CAD build for the part. Positions are in the model's coordinates, mm. A direction names the side the tool comes from. Coordinates: 2 decimals unless noted, no trailing zeros. Order: outer loops, then holes, each group sorted by start corner. A loop starts at its lowest first (then second) coordinate and runs counter-clockwise, first axis right, second up. Notation, with made-up numbers: M 0.5,-14 L 21.5,-14 A29 ccw 21.5,20 Z; hole C 23,27.5 d6. An arc over 180 degrees is marked long. Write item = value, one per line.
from build123d import *

# Parameters (mm, degrees)
BOSS_EXTRUDE1_DEPTH   = 6.35
FILLET1_R             = 5
F_6_CLEARANCE_HOLE1_D = 3.6576


with BuildPart() as part:
    # Sketch1 → Boss-Extrude1 (new body)
    with BuildSketch(Plane(origin=(0, 0, 0), x_dir=(0, 0, -1), z_dir=(1, 0, 0))):
        with BuildLine():
            Line((-27, -4), (-27, 4))
            Line((-27, 4), (-27, 9))
            ThreePointArc((-27, 9), (-22, 14), (-17, 9))
            Line((-17, 9), (-17, 4))
            Line((-17, 4), (17, 4))
            Line((17, 4), (17, 9))
            ThreePointArc((17, 9), (22, 14), (27, 9))
            Line((27, 9), (27, 4))
            Line((27, 4), (27, -4))
            Line((27, -4), (-27, -4))
        make_face()
    extrude(amount=BOSS_EXTRUDE1_DEPTH)

    # Fillet1
    fillet1_edges = [part.edges().sort_by_distance(p)[0] for p in [
        (3.175, -4, -27),
        (3.175, -4, 27),
    ]]
    fillet(fillet1_edges, radius=FILLET1_R)

    # #6 Clearance Hole1 (through all)
    with Locations(Plane.ZY):
        with Locations((-22, 9), (22, 9)):
            Hole(F_6_CLEARANCE_HOLE1_D / 2)


solid = part.part
(1) Slice it at D-D, the plane y = 11.75. Write the cut outline in (x, z).
Evaluation:
outline = M 0,-26.18 L 6.35,-26.18 L 6.35,-17.82 L 0,-17.82 Z; M 0,17.82 L 6.35,17.82 L 6.35,26.18 L 0,26.18 Z
(2) Slice it at B-B, the plane x = 1.5. Write the cut outline in (y, z), then the cut area to 3 significant figures.
Evaluation:
outline = M -4,-22 A5 ccw 1,-27 L 9,-27 A5 ccw 9,-17 L 4,-17 L 4,17 L 9,17 A5 ccw 9,27 L 1,27 A5 ccw -4,22 Z; hole C 9,-22 d3.66; hole C 9,22 d3.66
area = 579 mm²
(3) Pull direction Z, two halves, no side cores. Call faces 3 (the face through (3, -4, 0)), 4 (the face through (3, -2, -26)), 5 (the face through (3, 6, -17)): +Z half, -Z half, draft (parallel to the pull), parting line (faces both ways), or undercut.
Evaluation:
face_3 = draft
face_4 = -Z half
face_5 = undercut
(4) Slice it at C-C, the plane z = -9. Write the cut outline in (x, y), then the cut area to 3 significant figures.
Evaluation:
outline = M 0,-4 L 6.35,-4 L 6.35,4 L 0,4 Z
area = 50.8 mm²
(5) Slice it at A-A, the plane y = 4.5. Write the cut outline in (x, z).
Evaluation:
outline = M 0,-27 L 6.35,-27 L 6.35,-17 L 0,-17 Z; M 0,17 L 6.35,17 L 6.35,27 L 0,27 Z
(6) Wall check: line 1 (Y direction, x = 3, z = 22); line 2 (Z direction, x = 4.75, y = 9.75); line 3 (Z direction, x = 3.5, y = 7.75). Give the ranges that are in metal, low to high. Write a range as from..to.
Evaluation:
line_1 = -4..7.17, 10.83..14
line_2 = -26.94..-23.67, -20.33..-17.06, 17.06..20.33, 23.67..26.94
line_3 = -27..-23.33, -20.67..-17, 17..20.67, 23.33..27
(7) Tool access for faces 1 (the face through (3.22, 8.3, -23.69)), 2 (the face through (3, 4, 0)): list every direction of +Z, -Z, +X, -X, +Y, -Y with a clear straight run to the whole face (end or side of a thin tool).
Evaluation:
face_1 = +X, -X
face_2 = +X, -X, +Y
(8) Pin check, flat tip, straight feed: pin 1 Ø3 at (y, z) = (9, 22) entering from +X. Stop position of the tip, or through.
Evaluation:
pin_1 = through
